Geometry check sheet. Reference: the model listing, model coordinates, mm. Round coordinates to 2 decimals unless told otherwise and drop trailing zeros. Order: outer loops, then holes, each group sorted by start corner. A loop starts at its lowest first (then second) coordinate and runs counter-clockwise, first axis right, second up. Notation, with made-up numbers: (29.5, 64.25) -> (50.5, 64.25) arc R18 cw to (50.5, 75.25) -> close; hole circle Ø2 at (29.5, 34.25). An arc over 180 degrees is marked (long way). Use a Markdown table: item, result. Add a question column.
Item 1: Sectioned sample at A-A, the plane y = 0. Record the cut outline in (x, z), and give its area (3 significant figures).
Item 2: Material ranges on probe 1 along Y at (x, z) = (-9.65, -4.5); probe 2 along X at (y, z) = (19, -0.9); probe 3 along X at (y, z) = (40, -2.9), recorded low to high. Write a range as [from, to].
Item 3: Sectioned sample at D-D, the plane x = -19.5. Record the cut outline in (y, z).
Item 4: Gauge pin test, flat ends, axial feed: pin 1 Ø3.5 at (x, y) = (0, 9.65) entering from +Z; pin 2 Ø1 at (y, z) = (36, -3.5) entering from +X. Record the tip position at first contact, or that the pin passes through.
Item 5: Sectioned sample at B-B, the plane x = 9.65. Record the cut outline in (y, z), and give its area (3 significant figures).
Item 6: Sectioned sample at C-C, the plane z = -2.5. Record the cut outline in (x, y), and give its area (3 significant figures).
from build123d import *

# Parameters (mm, degrees)
ESQUISSE1_R        = 54
ESQUISSE1_R_2      = 2
ESQUISSE1_R_3      = 3.175
BOSS_EXTRU_1_DEPTH = 5.75
CUT_EXTRUDE1_REACH = 78.584
SKETCH1_R          = 6.35


with BuildPart() as part:
    # Esquisse1 → Boss.-Extru.1 (new body)
    with BuildSketch(Plane.XY):
        Circle(ESQUISSE1_R)
        with Locations((0, -9.65)):
            Circle(ESQUISSE1_R_2, mode=Mode.SUBTRACT)
        with Locations((0, 9.65)):
            Circle(ESQUISSE1_R_2, mode=Mode.SUBTRACT)
        with Locations((-9.65, 0)):
            Circle(ESQUISSE1_R_2, mode=Mode.SUBTRACT)
        with Locations((9.65, 0)):
            Circle(ESQUISSE1_R_2, mode=Mode.SUBTRACT)
        Circle(ESQUISSE1_R_3, mode=Mode.SUBTRACT)
    extrude(amount=-BOSS_EXTRU_1_DEPTH)

    # Sketch1 → Cut-Extrude1 (cut, up to next)
    with BuildSketch(Plane(origin=(0, 0, -5.75), x_dir=(-1, 0, 0), z_dir=(0, 0, -1)), mode=Mode.PRIVATE) as cut_extrude1_sk1:
        Circle(SKETCH1_R)
    cut_extrude1_tool1 = extrude(cut_extrude1_sk1.sketch, amount=-CUT_EXTRUDE1_REACH, mode=Mode.PRIVATE) & part.part
    add(cut_extrude1_tool1.solids().sort_by_distance((0, 0, -5.75))[0], mode=Mode.SUBTRACT)


solid = part.part
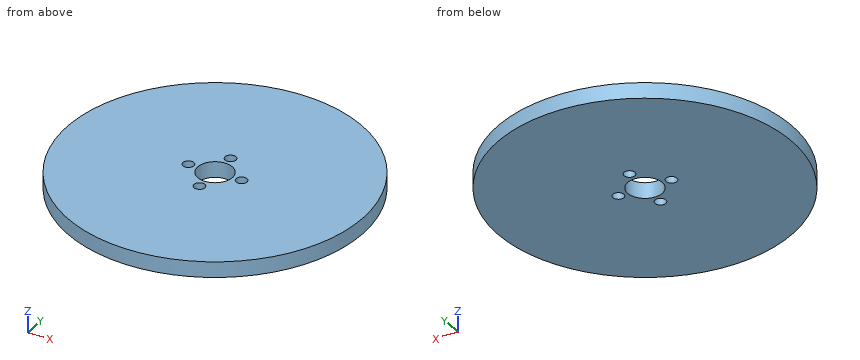
Found:
| question | item | result |
|---|---|---|
| 1 | outline | (-54, -5.75) -> (-11.65, -5.75) -> (-11.65, 0) -> (-54, 0) -> close; (-7.65, -5.75) -> (-6.35, -5.75) -> (-6.35, 0) -> (-7.65, 0) -> close; (6.35, -5.75) -> (7.65, -5.75) -> (7.65, 0) -> (6.35, 0) -> close; (11.65, -5.75) -> (54, -5.75) -> (54, 0) -> (11.65, 0) -> close |
| 1 | area | 502 mm2 |
| 2 | probe 1 | y = [-53.13, -2], [2, 53.13] |
| 2 | probe 2 | x = [-50.55, 50.55] |
| 2 | probe 3 | x = [-36.28, 36.28] |
| 3 | outline | (-50.36, -5.75) -> (50.36, -5.75) -> (50.36, 0) -> (-50.36, 0) -> close |
| 4 | pin 1 | passes through |
| 4 | pin 2 | stops at x = 40.69 |
| 5 | outline | (-53.13, -5.75) -> (-2, -5.75) -> (-2, 0) -> (-53.13, 0) -> close; (2, -5.75) -> (53.13, -5.75) -> (53.13, 0) -> (2, 0) -> close |
| 5 | area | 588 mm2 |
| 6 | outline | circle Ø108 at (0, 0); hole circle Ø4 at (-9.65, 0); hole circle Ø12.7 at (0, 0); hole circle Ø4 at (0, -9.65); hole circle Ø4 at (0, 9.65); hole circle Ø4 at (9.65, 0) |
| 6 | area | 8,980 mm2 |
